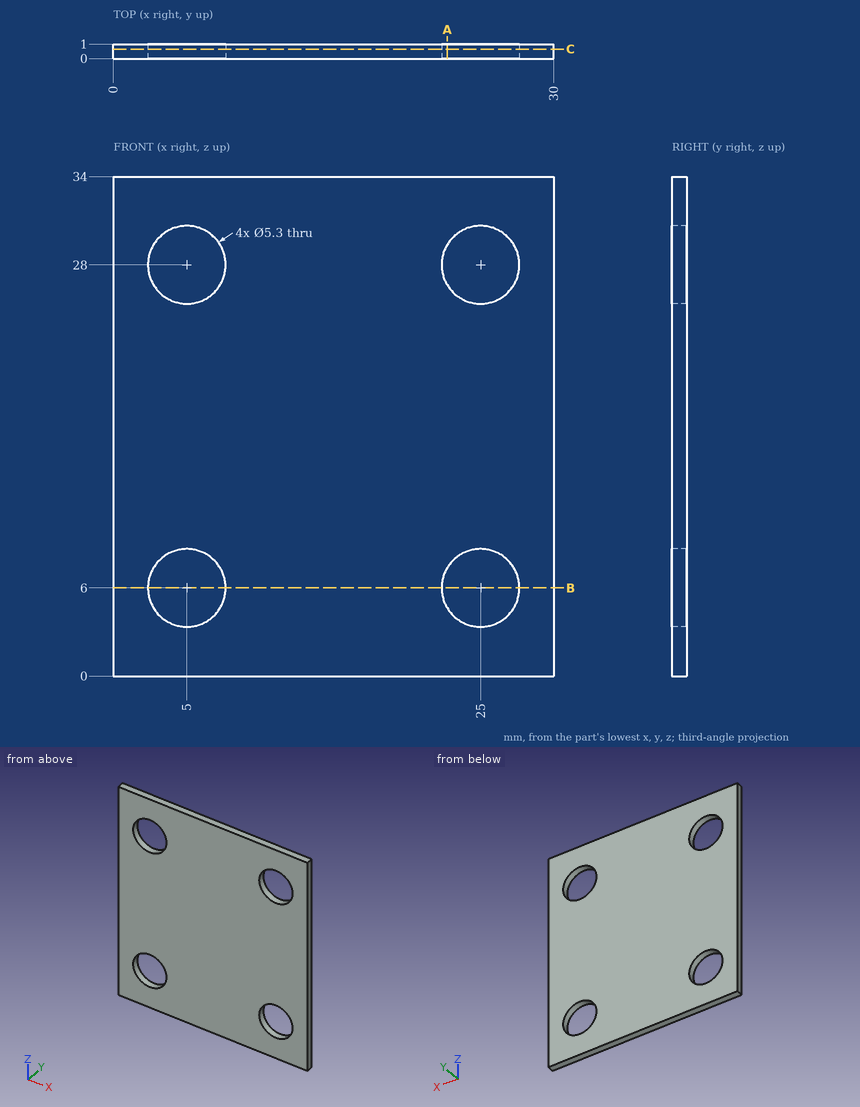
The drawing under review shows one solid part. Ordinate dimensions are in mm from its lowest x, y, z. Round coordinates to 2 decimals unless told otherwise and drop trailing zeros. Write each loop counter-clockwise with the first axis right and the second up, starting at its lowest first coordinate (ties: lowest second). Pieces come first, ordered by that corner, then holes. Notation, with made-up numbers: (14.5, 29.5) - (35.5, 29.5) arc R21 ccw to (35.5, 58.5) - close; hole circle Ø9 at (-33.75, -5). An arc over 180 degrees is marked (long way). Use one line per item in the form item = value.
Q1. Consider section A-A (x = 22.75). State the section outline as (y, z) points, and give its area (3 significant figures).
Answer key:
outline = (0, 0) - (1, 0) - (1, 4.6) - (0, 4.6) - close; (0, 7.4) - (1, 7.4) - (1, 26.6) - (0, 26.6) - close; (0, 29.4) - (1, 29.4) - (1, 34) - (0, 34) - close
area = 28.4 mm2
Q2. Consider section B-B (z = 6). State the section outline as (x, y) points, and give its area (3 significant figures).
Answer key:
outline = (0, 0) - (2.35, 0) - (2.35, 1) - (0, 1) - close; (7.65, 0) - (22.35, 0) - (22.35, 1) - (7.65, 1) - close; (27.65, 0) - (30, 0) - (30, 1) - (27.65, 1) - close
area = 19.4 mm2
Q3. For line 1 (X direction, y = 0.7, z = 28); line 2 (Z direction, x = 25, y = 0.7); line 3 (Z direction, x = 26, y = 0.9), list the stretches that pass through material, from the lowest coordinate up. Write a range as [from, to].
Answer key:
line_1 = [0, 2.35], [7.65, 22.35], [27.65, 30]
line_2 = [0, 3.35], [8.65, 25.35], [30.65, 34]
line_3 = [0, 3.55], [8.45, 25.55], [30.45, 34]
Q4. Insertion check: pin 1 Ø4 at (x, z) = (25, 28) entering from +Y. The pin has a flat end and moves straight along its axis. Give the tip position at first contact, or say it passes through.
Answer key:
pin_1 = through
Q5. Consider section C-C (y = 0.65). State the section outline as (x, z) points.
Answer key:
outline = (0, 0) - (30, 0) - (30, 34) - (0, 34) - close; hole circle Ø5.3 at (5, 6); hole circle Ø5.3 at (5, 28); hole circle Ø5.3 at (25, 6); hole circle Ø5.3 at (25, 28)
